The model under review builds one solid part; all positions refer to its coordinate system, in mm. A direction names the side the tool comes from. Coordinates: 2 decimals unless noted, no trailing zeros. Write each loop counter-clockwise with the first axis right and the second up, starting at its lowest first coordinate (ties: lowest second). Pieces come first, ordered by that corner, then holes. Notation, with made-up numbers: (42, -23.5) -> (99, -23.5) arc R13 cw to (99, -4.5) -> close; hole circle Ø11 at (31, 88). An arc over 180 degrees is marked (long way). Put each result on its own line as item: value. Start each with the question number.
from build123d import *

# Parameters (mm, degrees)
SKETCH1_W            = 152.4
SKETCH1_H            = 114.3
BOSS_EXTRUDE1_DEPTH  = 3.175
SKETCH2_W            = 152.4
SKETCH2_H            = 3.175
BOSS_EXTRUDE2_DEPTH  = 406.4
FILLET1_R            = 2.54
FILLET2_R            = 5.08
SKETCH3_R            = 30.988
SKETCH3_R_2          = 2.54
SKETCH3_R_3          = 2.159
SKETCH3_R_4          = 2.15
CUT_EXTRUDE1_DEPTH   = 418.41289211
CONVERT_SOLID1_START = -76.2
CONVERT_SOLID1_DEPTH = 152.4
SKETCH4_R            = 4.7625
SKETCH4_R_2          = 4.826
CUT_EXTRUDE2_DEPTH   = 432.169208374


# Read off the part's stored shape, not the designer's step: Convert-Solid1
with BuildPart() as part:
    # Sketch1 → Boss-Extrude1 (new body)
    with BuildSketch(Plane(origin=(0, 0, 0), x_dir=(1, 0, 0), z_dir=(0, 1, 0))):
        Rectangle(SKETCH1_W, SKETCH1_H)
    extrude(amount=BOSS_EXTRUDE1_DEPTH)

    # Sketch2 → Boss-Extrude2 (add)
    with BuildSketch(Plane(origin=(0, 3.175, 0), x_dir=(1, 0, 0), z_dir=(0, 1, 0))):
        with Locations((0, -55.5625)):
            Rectangle(SKETCH2_W, SKETCH2_H)
    extrude(amount=BOSS_EXTRUDE2_DEPTH)

    # Fillet1
    fillet1_edges = [part.edges().sort_by_distance(p)[0] for p in [
        (0, 3.175, 53.975),
        (0, 0, 57.15),
    ]]
    fillet(fillet1_edges, radius=FILLET1_R)

    # Fillet2
    fillet2_edges = [part.edges().sort_by_distance(p)[0] for p in [
        (-76.2, 409.575, 55.5625),
        (76.2, 409.575, 55.5625),
        (-76.2, 1.5875, -57.15),
        (76.2, 1.5875, -57.15),
    ]]
    fillet(fillet2_edges, radius=FILLET2_R)

    # Sketch3 → Cut-Extrude1 (cut, through all)
    with BuildSketch(Plane(origin=(0, 3.175, 0), x_dir=(1, 0, 0), z_dir=(0, 1, 0))):
        with Locations(Location((-25.4, 3.81, 0), (0, 0, 270))):
            Circle(SKETCH3_R)
        with Locations(Location((15.875, 44.958, 0), (0, 0, 270))):
            Circle(SKETCH3_R_2)
        with Locations(Location((-66.675, -37.465, 0), (0, 0, 270))):
            Circle(SKETCH3_R_2)
        with Locations(Location((15.875, -37.465, 0), (0, 0, 270))):
            Circle(SKETCH3_R_2)
        with Locations(Location((30.988, 44.45, 0), (0, 0, 270))):
            Circle(SKETCH3_R_3)
        with Locations(Location((60.93860251, 44.46, 0), (0, 0, 270))):
            Circle(SKETCH3_R_4)
        with Locations(Location((60.96, 14.478, 0), (0, 0, 270))):
            Circle(SKETCH3_R_3)
        with Locations(Location((30.93860251, 14.478, 0), (0, 0, 270))):
            Circle(SKETCH3_R_3)
        with Locations(Location((-66.675, 45.085, 0), (0, 0, 270))):
            Circle(SKETCH3_R_2)
    extrude(amount=-CUT_EXTRUDE1_DEPTH, mode=Mode.SUBTRACT)

    # Convert-Solid1 outline → Convert-Solid1 (cut)
    with BuildSketch(Plane.YZ.offset(CONVERT_SOLID1_START)):
        with BuildLine():
            Line((1.5875, -57.15), (1.5875, 51.435))
            ThreePointArc((1.5875, 51.435), (2.796416761, 54.353583239), (5.715, 55.5625))
            Line((5.715, 55.5625), (409.575, 55.5625))
            Line((409.575, 55.5625), (409.575, 57.15))
            Line((409.575, 57.15), (2.54, 57.15))
            ThreePointArc((2.54, 57.15), (0.743948776, 56.406051224), (0, 54.61))
            Line((0, 54.61), (0, -57.15))
            Line((0, -57.15), (1.5875, -57.15))
        make_face()
    extrude(amount=CONVERT_SOLID1_DEPTH, mode=Mode.SUBTRACT)

    # Sketch4 → Cut-Extrude2 (cut, through all)
    with BuildSketch(Plane(origin=(0, 0, 53.975), x_dir=(-1, 0, 0), z_dir=(0, 0, -1))):
        with Locations((-44.45, 390.525)):
            Circle(SKETCH4_R)
        with Locations((44.45, 390.525)):
            Circle(SKETCH4_R)
        with Locations((-44.45, 183.515)):
            Circle(SKETCH4_R_2)
        with Locations((44.45, 37.465)):
            Circle(SKETCH4_R_2)
    extrude(amount=-CUT_EXTRUDE2_DEPTH, mode=Mode.SUBTRACT)


solid = part.part
1. Consider section C-C on z = -3.81. State the section outline as (x, y) points (1 decimal).
2. Consider section B-B on x = 44.45. State how many separate pieces and enclosed holes the cut face has, then the cut area to 3 significant figures.
3. Insertion check: P1, Ø1.5, axis at x = -43.5, y = 367.5, coming from the -Z side (3 decimals); P2, Ø12, axis at x = 58.5, z = 2, coming from the +Y side (3 decimals); P3, Ø5, axis at x = 60.94, z = -44.46, coming from the -Y side. Each pin has a flat end and moves straight along its axis. Give the tip position at first contact, or say it passes through.
4. Wall thickness on line 1 (X direction, y = 2.45, z = -44.46); line 2 (Y direction, x = 12, z = 44.5) (1 decimal); line 3 (Z direction, x = -65.5, y = 110.5) (1 decimal): over which ranges is each line inside the solid? List them lowest first. Write a range as from..to.
5. Tool access review of faces 3 (the flat face through (-1, 205, 55.562)), 4 (the flat face through (16, 3.175, -4)): name each direction out of +Z, -Z, +X, -X, +Y, -Y from which nothing blocks a thin tool from reaching the whole face with its end or side.
6. The part is to be moulded in two halves that separate along X. For faces 1 (the flat face through (-1, 205, 53.975)), 2 (the cylindrical face through (-39.63, 37.68, 54.76)), say which applies: released by +X, released by -X, zero draft, split by the parting line, or undercut.
Output values:
1. outline: (-76.2, 1.6) -> (-56.4, 1.6) -> (-56.4, 3.2) -> (-76.2, 3.2) -> close; (5.6, 1.6) -> (76.2, 1.6) -> (76.2, 3.2) -> (5.6, 3.2) -> close
2. separate pieces: 3
2. enclosed holes: 0
2. area: 791 mm^2
3. P1: stops at z = 53.975
3. P2: stops at y = 3.175
3. P3: stops at y = 1.59
4. line 1: x = -76.2..-69.14, -64.21..13.38, 18.37..28.83, 33.15..58.79, 63.09..76.2
4. line 2: y = 1.6..3.2
4. line 3: z = 54..55.6
5. face 3: +Z, +X, -X, +Y, -Y
5. face 4: -Z, +X, -X, +Y
6. face 1: zero draft
6. face 2: undercut
